The model under review builds one solid part; all positions refer to its coordinate system, in mm. A direction names the side the tool comes from. Round coordinates to 2 decimals unless told otherwise and drop trailing zeros. Order: outer loops, then holes, each group sorted by start corner. A loop starts at its lowest first (then second) coordinate and runs counter-clockwise, first axis right, second up. Notation, with made-up numbers: M -25.5,30 L 16.5,30 A17 cw 16.5,55 Z; hole C -30,-28.5 d8. An arc over 180 degrees is marked long. One line per item, written item: value. Start each with the question number.
from build123d import *

# Parameters (mm, degrees)
BASE_FLANGE1_DEPTH             = 1050
CUT_EXTRUDE1_REACH             = 1056.479
EDGE_FLANGE5_STRIP_W           = 20
EDGE_FLANGE5_STRIP_H           = 1
EDGE_FLANGE5_STRIP_CUT_DEPTH   = 52
EDGE_FLANGE5_STRIP_2_W         = 20
EDGE_FLANGE5_STRIP_2_H         = 1
EDGE_FLANGE5_STRIP_CUT_2_DEPTH = 12
EDGE_FLANGE5_DEPTH             = 52
EDGE_FLANGE5_BEND_DEPTH        = 12
EDGE_FLANGE7_DEPTH             = 1046
EDGE_FLANGE8_STRIP_W           = 10
EDGE_FLANGE8_STRIP_H           = 1
EDGE_FLANGE8_STRIP_CUT_DEPTH   = 12
EDGE_FLANGE8_DEPTH             = 12
EDGE_FLANGE9_START             = 529.5
EDGE_FLANGE9_DEPTH             = 515.5
EDGE_FLANGE9_2_DEPTH           = 0.5
EDGE_FLANGE9_START_2           = 530
EDGE_FLANGE9_3_DEPTH           = 515


# Read off the part's stored shape, not the designer's step: Edge-Flange9
# Sheet-metal steps are written as plain solids
with BuildPart() as part:
    # Sketch1 → Base-Flange1 (new body)
    with BuildSketch(Plane(origin=(0, 0, 0), x_dir=(1, 0, 0), z_dir=(0, 1, 0))):
        with BuildLine():
            Line((0, 0), (-12, 0))
            ThreePointArc((-12, 0), (-14.121320344, -0.878679656), (-15, -3))
            Line((-15, -3), (-15, -16))
            ThreePointArc((-15, -16), (-16.171572875, -18.828427125), (-19, -20))
            Line((-19, -20), (-31, -20))
            ThreePointArc((-31, -20), (-33.828427125, -18.828427125), (-35, -16))
            Line((-35, -16), (-35, -3))
            ThreePointArc((-35, -3), (-35.878679656, -0.878679656), (-38, 0))
            Line((-38, 0), (-95, 0))
            Line((-95, 0), (-95, 1))
            Line((-95, 1), (-38, 1))
            ThreePointArc((-38, 1), (-35.171572875, -0.171572875), (-34, -3))
            Line((-34, -3), (-34, -16))
            ThreePointArc((-34, -16), (-33.121320344, -18.121320344), (-31, -19))
            Line((-31, -19), (-19, -19))
            ThreePointArc((-19, -19), (-16.878679656, -18.121320344), (-16, -16))
            Line((-16, -16), (-16, -3))
            ThreePointArc((-16, -3), (-14.828427125, -0.171572875), (-12, 1))
            Line((-12, 1), (0, 1))
            Line((0, 1), (0, 0))
        make_face()
    extrude(amount=BASE_FLANGE1_DEPTH)

    # Sketch18 → Cut-Extrude1 (cut, up to next)
    with BuildSketch(Plane.XY, mode=Mode.PRIVATE) as cut_extrude1_sk1:
        with BuildLine():
            Line((-95, 1045), (-95, 1050))
            Line((-95, 1050), (-90, 1050))
            ThreePointArc((-90, 1050), (-93.535533906, 1048.535533906), (-95, 1045))
        make_face()
    cut_extrude1_tool1 = extrude(cut_extrude1_sk1.sketch, amount=-CUT_EXTRUDE1_REACH, mode=Mode.PRIVATE) & part.part
    add(cut_extrude1_tool1.solids().sort_by_distance((-93.88316, 1048.88316, 0))[0], mode=Mode.SUBTRACT)

    # Edge-Flange5 strip (across the edge) → Edge-Flange5 strip cut (cut)
    with BuildSketch(Plane(origin=(-90, 1050, -1), x_dir=(0, -1, 0), z_dir=(1, 0, 0))):
        with Locations((-6, -0.5)):
            Rectangle(EDGE_FLANGE5_STRIP_W, EDGE_FLANGE5_STRIP_H)
    extrude(amount=EDGE_FLANGE5_STRIP_CUT_DEPTH, mode=Mode.SUBTRACT)

    # Edge-Flange5 strip 2 (across the edge) → Edge-Flange5 strip cut 2 (cut)
    with BuildSketch(Plane(origin=(-12, 1050, -1), x_dir=(0, -1, 0), z_dir=(1, 0, 0))):
        with Locations((-6, -0.5)):
            Rectangle(EDGE_FLANGE5_STRIP_2_W, EDGE_FLANGE5_STRIP_2_H)
    extrude(amount=EDGE_FLANGE5_STRIP_CUT_2_DEPTH, mode=Mode.SUBTRACT)

    # Edge-Flange5 section (across the edge) → Edge-Flange5 (add)
    with BuildSketch(Plane(origin=(-90, 1050, -1), x_dir=(0, -1, 0), z_dir=(1, 0, 0))):
        with BuildLine():
            Line((0, 3), (0, 19))
            Line((0, 19), (1, 19))
            Line((1, 19), (1, 3))
            ThreePointArc((1, 3), (1.878679656, 0.878679656), (4, 0))
            Line((4, 0), (4, -1))
            ThreePointArc((4, -1), (1.171572875, 0.171572875), (0, 3))
        make_face()
    extrude(amount=EDGE_FLANGE5_DEPTH)

    # Edge-Flange5 section 2 (across the edge) → Edge-Flange5 bend (add)
    with BuildSketch(Plane(origin=(-12, 1050, -1), x_dir=(0, -1, 0), z_dir=(1, 0, 0))):
        with BuildLine():
            Line((0, 3), (0, 19))
            Line((0, 19), (1, 19))
            Line((1, 19), (1, 3))
            ThreePointArc((1, 3), (1.878679656, 0.878679656), (4, 0))
            Line((4, 0), (4, -1))
            ThreePointArc((4, -1), (1.171572875, 0.171572875), (0, 3))
        make_face()
    extrude(amount=EDGE_FLANGE5_BEND_DEPTH)

    # Edge-Flange7 section (across the edge) → Edge-Flange7 (add)
    with BuildSketch(Plane(origin=(3, 1046, -1), x_dir=(-1, 0, 0), z_dir=(0, -1, 0))):
        with BuildLine():
            Line((-1, 3), (-1, 29))
            Line((-1, 29), (0, 29))
            Line((0, 29), (0, 3))
            ThreePointArc((0, 3), (0.878679656, 0.878679656), (3, 0))
            Line((3, 0), (3, -1))
            ThreePointArc((3, -1), (0.171572875, 0.171572875), (-1, 3))
        make_face()
    extrude(amount=EDGE_FLANGE7_DEPTH)

    # Edge-Flange8 strip (across the edge) → Edge-Flange8 strip cut (cut)
    with BuildSketch(Plane(origin=(-31, 1050, 19), x_dir=(0, -1, 0), z_dir=(1, 0, 0))):
        with Locations((-1, -0.5)):
            Rectangle(EDGE_FLANGE8_STRIP_W, EDGE_FLANGE8_STRIP_H)
    extrude(amount=EDGE_FLANGE8_STRIP_CUT_DEPTH, mode=Mode.SUBTRACT)

    # Edge-Flange8 section (across the edge) → Edge-Flange8 (add)
    with BuildSketch(Plane(origin=(-31, 1050, 19), x_dir=(0, -1, 0), z_dir=(1, 0, 0))):
        with BuildLine():
            Line((0, 3), (0, 29))
            Line((0, 29), (1, 29))
            Line((1, 29), (1, 3))
            ThreePointArc((1, 3), (1.878679656, 0.878679656), (4, 0))
            Line((4, 0), (4, -1))
            ThreePointArc((4, -1), (1.171572875, 0.171572875), (0, 3))
        make_face()
    extrude(amount=EDGE_FLANGE8_DEPTH)

    # Edge-Flange9 outline → Edge-Flange9 (cut)
    with BuildSketch(Plane(origin=(0, 0, 0), x_dir=(1, 0, 0), z_dir=(0, 1, 0)).offset(EDGE_FLANGE9_START)):
        with BuildLine():
            ThreePointArc((-91, 0), (-92.414213563, 0.258342613), (-93.645751312, 1))
            Line((-93.645751312, 1), (-95, 1))
            Line((-95, 1), (-95, 0))
            Line((-95, 0), (-91, 0))
        make_face()
    extrude(amount=EDGE_FLANGE9_DEPTH, mode=Mode.SUBTRACT)

    # Edge-Flange9 2 outline → Edge-Flange9 2 (cut)
    with BuildSketch(Plane(origin=(0, 0, 0), x_dir=(1, 0, 0), z_dir=(0, 1, 0)).offset(EDGE_FLANGE9_START)):
        with BuildLine():
            Line((-90.5, 1), (-93.645751312, 1))
            ThreePointArc((-93.645751312, 1), (-92.414213563, 0.258342613), (-91, 0))
            Line((-91, 0), (-90.5, 0))
            Line((-90.5, 0), (-90.5, 1))
        make_face()
    extrude(amount=EDGE_FLANGE9_2_DEPTH, mode=Mode.SUBTRACT)

    # Edge-Flange9 3 outline → Edge-Flange9 3 (add)
    with BuildSketch(Plane(origin=(0, 0, 0), x_dir=(1, 0, 0), z_dir=(0, 1, 0)).offset(EDGE_FLANGE9_START_2)):
        with BuildLine():
            Line((-95, 21), (-95, 4))
            ThreePointArc((-95, 4), (-94.645751311, 2.354248689), (-93.645751312, 1))
            Line((-93.645751312, 1), (-91, 1))
            ThreePointArc((-91, 1), (-93.121320344, 1.878679656), (-94, 4))
            Line((-94, 4), (-94, 21))
            Line((-94, 21), (-95, 21))
        make_face()
    extrude(amount=EDGE_FLANGE9_3_DEPTH)


with BuildPart() as body_2:
    # Mirror5: mirrored copy
    add(part.part.mirror(Plane.XY.offset(40)))


solid = body_2.part
Item 1: Consider section C-C, the plane y = 646.5. Give the boundary of the cut face in (x, z).
Item 2: Wall thickness on L1, parallel to X at y = 886.5, z = 77; L2, parallel to X at y = 249, z = 63; L3, parallel to Z at x = -54.5, y = 775.5: over which ranges is each line inside the solid? List them lowest first.
Item 3: Machinability: for faces 4 (the flat face through (-64, 1049, 92)), 5 (the flat face through (-94, 784, 92)), 6 (the flat face through (-95, 784, 93)), which of the approach directions +Z, -Z, +X, -X, +Y, -Y give a long, thin tool a straight path to every point of the face, cutting with its end or side? Answer none if there is none.
Item 4: Consider section A-A, the plane y = 209. Give the boundary of the cut face in (x, z), then the cut area to 3 significant figures.
Item 5: Consider section B-B, the plane x = -60. Give the boundary of the cut face in (y, z).
Item 6: The part is to be moulded in two halves that separate along X. For faces 1 (the flat face through (-66, 518, 80)), 2 (the flat face through (-67, 518, 81)), 3 (the flat face through (4, 530, 97)), say which applies: pulls with the +X half, pulls with the -X half, needs draft (parallel to the pull), parting line crosses it, or undercut.
Item 7: Clearance check with flat-ended pins moving along their axes: P1, Ø0.8, axis at y = 1048, z = 60.5, coming from the +X side; P2, Ø4.5, axis at y = 1047, z = 93, coming from the -X side; P3, Ø13, axis at x = -27, y = 316.5, coming from the +Z side; P4, Ø3, axis at y = 1048, z = 70, coming from the -X side. State where each tip first meets the part, or that it passes through.
Computed:
1. outline: M -95,84 A4 ccw -91,80 L -38,80 A3 cw -35,77 L -35,64 A4 ccw -31,60 L -19,60 A4 ccw -15,64 L -15,77 A3 cw -12,80 L 0,80 A4 ccw 4,84 L 4,110 L 3,110 L 3,84 A3 cw 0,81 L -12,81 A4 ccw -16,77 L -16,64 A3 cw -19,61 L -31,61 A3 cw -34,64 L -34,77 A4 ccw -38,81 L -91,81 A3 cw -94,84 L -94,101 L -95,101 Z
2. L1: x = -35 to -34, -16 to -15
2. L2: x = -34.87 to -33.83, -16.17 to -15.13
2. L3: z = 80 to 81
3. face 4: +Z, +X, -X, -Y
3. face 5: +Z, +Y, -Y
3. face 6: +Z, -Z, -X, +Y, -Y
4. outline: M -95,80 L -38,80 A3 cw -35,77 L -35,64 A4 ccw -31,60 L -19,60 A4 ccw -15,64 L -15,77 A3 cw -12,80 L 0,80 A4 ccw 4,84 L 4,110 L 3,110 L 3,84 A3 cw 0,81 L -12,81 A4 ccw -16,77 L -16,64 A3 cw -19,61 L -31,61 A3 cw -34,64 L -34,77 A4 ccw -38,81 L -95,81 Z
4. area: 160 mm^2
5. outline: M 0,80 L 1046,80 A4 ccw 1050,84 L 1050,100 L 1049,100 L 1049,84 A3 cw 1046,81 L 0,81 Z
6. face 1: needs draft
6. face 2: undercut
6. face 3: pulls with the +X half
7. P1: stops at x = -16.47
7. P2: stops at x = -95
7. P3: stops at z = 62.34
7. P4: stops at x = -35
